Check sheet for the modelled part. Datum: model origin and axes. Units: mm. Face numbers are marked on the shaded views. A direction names the side the tool comes from. Coordinates: 2 decimals unless noted, no trailing zeros. Write each loop counter-clockwise with the first axis right and the second up, starting at its lowest first coordinate (ties: lowest second). Pieces come first, ordered by that corner, then holes. Notation, with made-up numbers: (22.5, 65) - (29.5, 65) arc R23 cw to (29.5, 104) - close; hole circle Ø1 at (62, -7.75). An arc over 180 degrees is marked (long way). Write each question's results on one line, items separated by ' | '.
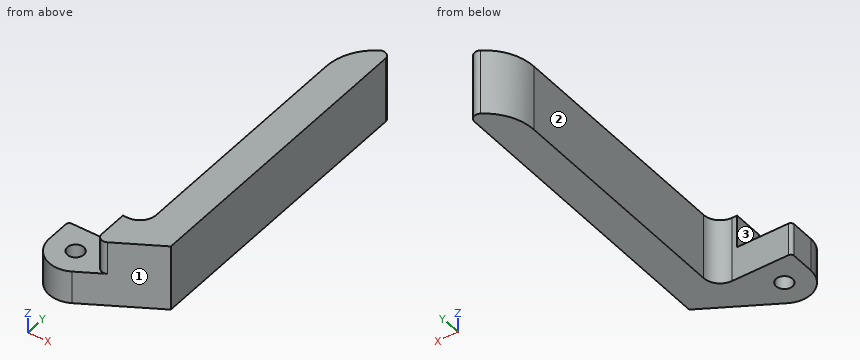
from build123d import *

# Parameters (mm, degrees)
SKETCH1_R           = 2.5
BOSS_EXTRUDE1_DEPTH = 20
CUT_EXTRUDE1_DEPTH  = 10


with BuildPart() as part:
    # Sketch1 → Boss-Extrude1 (new body)
    with BuildSketch(Plane.XY):
        with BuildLine():
            Line((-7, 8), (10, 8))
            ThreePointArc((10, 8), (13.535533906, 9.464466094), (15, 13))
            Line((15, 13), (15, 83.857864376))
            ThreePointArc((15, 83.857864376), (16.84412971, 91.063631297), (21.923076923, 96.497615703))
            ThreePointArc((21.923076923, 96.497615703), (23.960768923, 96.566431565), (25, 94.812315526))
            Line((25, 94.812315526), (25, 5.196152423))
            Line((25, 5.196152423), (4, -6.92820323))
            ThreePointArc((4, -6.92820323), (-4, -6.92820323), (-8, 0))
            Line((-8, 0), (-8, 7))
            ThreePointArc((-8, 7), (-7.707106781, 7.707106781), (-7, 8))
        make_face()
        Circle(SKETCH1_R, mode=Mode.SUBTRACT)
    extrude(amount=BOSS_EXTRUDE1_DEPTH)

    # Sketch2 → Cut-Extrude1 (cut)
    with BuildSketch(Plane.XY.offset(20)):
        with BuildLine():
            Line((8.5, 8), (8.5, -0.866025404))
            ThreePointArc((8.5, -0.866025404), (9.5, -2.598076211), (11.5, -2.598076211))
            Line((11.5, -2.598076211), (4, -6.92820323))
            ThreePointArc((4, -6.92820323), (-4, -6.92820323), (-8, 0))
            Line((-8, 0), (-8, 7))
            ThreePointArc((-8, 7), (-7.707106781, 7.707106781), (-7, 8))
            Line((-7, 8), (8.5, 8))
        make_face()
    extrude(amount=-CUT_EXTRUDE1_DEPTH, mode=Mode.SUBTRACT)


solid = part.part
1. Material ranges on L1, parallel to Y at x = 0, z = 7.5; L2, parallel to X at y = 79.5, z = 12.75; L3, parallel to Y at x = -1, z = 6, recorded low to high. Write a range as [from, to].
Values follow:
L1: y = [-8, -2.5], [2.5, 8] | L2: x = [15, 25] | L3: y = [-7.94, -2.29], [2.29, 8]
2. Go/stop test with flat-tipped pins: pin 1 (10 mm diameter, centred on x = -1, y = 7, fed in from +Z); pin 2 (2.5 mm diameter, centred on y = 5, z = 14, fed in from -X); pin 3 (1 mm diameter, centred on y = 82, z = 8, fed in from -X); pin 4 (4 mm diameter, centred on x = 16.5, y = 38.5, fed in from -Z). Record where each tip stops, or that it passes through.
Values follow:
pin 1: stops at z = 10 | pin 2: stops at x = 8.5 | pin 3: stops at x = 15 | pin 4: stops at z = 0
3. Sectioned sample at B-B (z = 4). Record the cut outline in (x, y).
Values follow:
outline: (-8, 0) arc R8 ccw to (4, -6.93) - (25, 5.2) - (25, 94.81) arc R2 ccw to (21.92, 96.5) arc R15 ccw to (15, 83.86) - (15, 13) arc R5 cw to (10, 8) - (-7, 8) arc R1 ccw to (-8, 7) - close; hole circle Ø5 at (0, 0)
4. Access from +Z, -Z, +X, -X, +Y, -Y to the whole of each face (thin tool, end or side, straight path). Record for the marked faces 1, 2 and 3.
Values follow:
face 1: +Z, -Z, +X, -Y | face 2: +Z, -Z, -X, +Y | face 3: +Z, -X, +Y, -Y
5. Sectioned sample at D-D (z = 15). Record the cut outline in (x, y).
Values follow:
outline: (8.5, -0.87) arc R2 ccw to (11.5, -2.6) - (25, 5.2) - (25, 94.81) arc R2 ccw to (21.92, 96.5) arc R15 ccw to (15, 83.86) - (15, 13) arc R5 cw to (10, 8) - (8.5, 8) - close
6. Sectioned sample at C-C (y = 31.5). Record the cut outline in (x, z).
Values follow:
outline: (15, 0) - (25, 0) - (25, 20) - (15, 20) - close
7. Sectioned sample at A-A (x = 0). Record the cut outline in (y, z), then the cut area to 3 significant figures.
Values follow:
outline: (-8, 0) - (-2.5, 0) - (-2.5, 10) - (-8, 10) - close; (2.5, 0) - (8, 0) - (8, 10) - (2.5, 10) - close | area: 110 mm^2
